Part model, mm, in its own coordinate system. Give positions to 0.01 mm unless a question says otherwise; leave off trailing zeros. Order: outer loops, then holes, each group sorted by start corner. A loop starts at its lowest first (then second) coordinate and runs counter-clockwise, first axis right, second up. Notation, with made-up numbers: (78, 66) - (124, 66) arc R15 cw to (124, 75) - close; hole circle Ø4 at (62, 73.25). An arc over 180 degrees is marked (long way). Use a Markdown table: item, result. Add a question column.
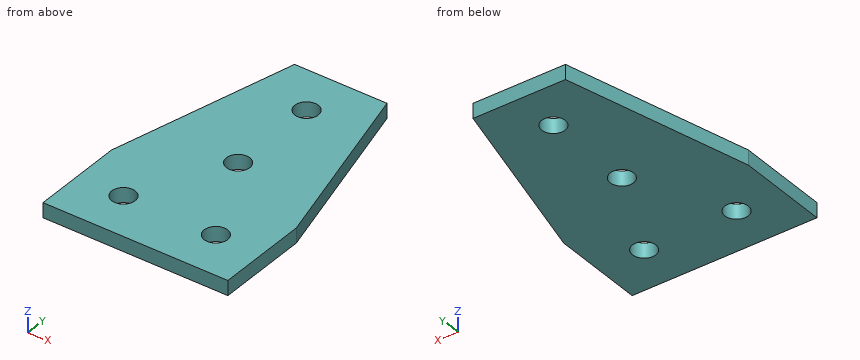
Autodesk Inventor part; units mm, degrees
ref_plane "YZ Plane" through (0, 0, 0) normal (1, 0, 0) x (0, 1, 0)
ref_plane "XZ Plane" through (0, 0, 0) normal (0, 1, 0) x (-1, 0, 0)
ref_plane "XY Plane" through (0, 0, 0) normal (0, 0, 1) x (1, 0, 0)
sketch "Sketch_1" plane through (0, 0, 0) normal (0, 0, 1) x (1, 0, 0)
  line L0 (-25, 25) -> (-25, 0)
  line L1 (-25, 0) -> (25, 0)
  line L2 (25, 0) -> (25, 25)
  line L3 (25, 25) -> (12.5, 75)
  line L4 (12.5, 75) -> (-12.5, 75)
  line L5 (-12.5, 75) -> (-25, 25)
  circle A0 centre (12.5, 12.5) radius 3.175
  circle A1 centre (0, 37.5) radius 3.175
  circle A2 centre (0, 62.5) radius 3.175
  circle A3 centre (-12.5, 12.5) radius 3.175
extrude "Extrusion1" add sketch "Sketch_1" along normal blind 4
properties part number "25-4141"
1. Cut at A-A (x = 0). Write the cut outline in (y, z) (3 decimals).
2. Cut at D-D (y = 62.5). Write the cut outline in (x, z) (3 decimals), plus the area to 3 significant figures.
3. Pin check, flat tip, straight feed: P1, Ø8.5, axis at x = 0, y = 62.5, coming from the +Z side. Stop position of the tip, or through.
4. Cut at B-B (z = 0.8). Write the cut outline in (x, y) (3 decimals), plus the area to 3 significant figures.
5. Cut at C-C (y = 12.5). Write the cut outline in (x, z) (3 decimals).
6. Drill centre lines: probe 1 along Y at (x, z) = (0, 2.4) (3 decimals); probe 2 along X at (y, z) = (11.5, 2); probe 3 along X at (y, z) = (39, 3.35). Where is each one in solid material? Low to high. Write a range as [from, to].
Responses:
| question | item | result |
|---|---|---|
| 1 | outline | (0, 0) - (34.325, 0) - (34.325, 4) - (0, 4) - close; (40.675, 0) - (59.325, 0) - (59.325, 4) - (40.675, 4) - close; (65.675, 0) - (75, 0) - (75, 4) - (65.675, 4) - close |
| 2 | outline | (-15.625, 0) - (-3.175, 0) - (-3.175, 4) - (-15.625, 4) - close; (3.175, 0) - (15.625, 0) - (15.625, 4) - (3.175, 4) - close |
| 2 | area | 99.6 mm² |
| 3 | P1 | stops at z = 4 |
| 4 | outline | (-25, 0) - (25, 0) - (25, 25) - (12.5, 75) - (-12.5, 75) - (-25, 25) - close; hole circle Ø6.35 at (-12.5, 12.5); hole circle Ø6.35 at (0, 37.5); hole circle Ø6.35 at (0, 62.5); hole circle Ø6.35 at (12.5, 12.5) |
| 4 | area | 3,000 mm² |
| 5 | outline | (-25, 0) - (-15.675, 0) - (-15.675, 4) - (-25, 4) - close; (-9.325, 0) - (9.325, 0) - (9.325, 4) - (-9.325, 4) - close; (15.675, 0) - (25, 0) - (25, 4) - (15.675, 4) - close |
| 6 | probe 1 | y = [0, 34.325], [40.675, 59.325], [65.675, 75] |
| 6 | probe 2 | x = [-25, -15.51], [-9.49, 9.49], [15.51, 25] |
| 6 | probe 3 | x = [-21.5, -2.8], [2.8, 21.5] |
